```python
from build123d import *

# Parameters (mm, degrees)
SKETCH1_R           = 3.556
BOSS_EXTRUDE2_DEPTH = 6.35
SKETCH2_W           = 25.4
SKETCH2_H           = 12.7
BOSS_EXTRUDE3_DEPTH = 8.255
SKETCH3_W           = 1.27
SKETCH3_H           = 3.175
CUT_EXTRUDE1_DEPTH  = 3.175
SKETCH4_R           = 6.477
CUT_EXTRUDE2_DEPTH  = 6.604
FILLET1_R           = 8.255


with BuildPart() as part:
    # Sketch1 → Boss-Extrude2 (new body)
    with BuildSketch(Plane(origin=(0, 0, 0), x_dir=(1, 0, 0), z_dir=(0, 1, 0))):
        with BuildLine():
            Line((-12.7, 0), (-12.7, 38.1))
            Line((-12.7, 38.1), (12.7, 38.1))
            Line((12.7, 38.1), (12.7, 0))
            ThreePointArc((12.7, 0), (0, -12.7), (-12.7, 0))
        make_face()
        Circle(SKETCH1_R, mode=Mode.SUBTRACT)
    extrude(amount=BOSS_EXTRUDE2_DEPTH)

    # Sketch2 → Boss-Extrude3 (add)
    with BuildSketch(Plane.XZ):
        with Locations((0, -31.75)):
            Rectangle(SKETCH2_W, SKETCH2_H)
    extrude(amount=BOSS_EXTRUDE3_DEPTH)

    # Sketch3 → Cut-Extrude1 (cut)
    with BuildSketch(Plane.XY.offset(-25.4)):
        with Locations((0, -4.7625)):
            Rectangle(SKETCH3_W, SKETCH3_H)
    extrude(amount=-CUT_EXTRUDE1_DEPTH, mode=Mode.SUBTRACT)

    # Sketch4 → Cut-Extrude2 (cut)
    with BuildSketch(Plane(origin=(0, 0, -38.1), x_dir=(-1, 0, 0), z_dir=(0, 0, -1))):
        with Locations((0, -0.9525)):
            Circle(SKETCH4_R)
    extrude(amount=-CUT_EXTRUDE2_DEPTH, mode=Mode.SUBTRACT)

    # Fillet1
    fillet1_edges = [part.edges().sort_by_distance(p)[0] for p in [
        (-12.7, -8.255, -31.75),
        (12.7, -8.255, -31.75),
    ]]
    fillet(fillet1_edges, radius=FILLET1_R)


solid = part.part
```
CAD build for the part. Positions are in the model's coordinates, mm. A direction names the side the tool comes from. Round coordinates to 2 decimals unless told otherwise and drop trailing zeros. Order: outer loops, then holes, each group sorted by start corner. A loop starts at its lowest first (then second) coordinate and runs counter-clockwise, first axis right, second up. Notation, with made-up numbers: (-20.75, 46.5) -> (-10.75, 46.5) arc R9 cw to (-10.75, 60.5) -> close; hole circle Ø4 at (-16, -6). An arc over 180 degrees is marked (long way). Write item = value, one per line.
(1) Drill centre lines: L1, parallel to Y at x = 0.5, z = 4.5; L2, parallel to Z at x = -1.25, y = -2; L3, parallel to Z at x = 1, y = 5.5. Where is each one in solid material? Low to high.
Answers follow:
L1 = 0 to 6.35
L2 = -31.5 to -25.4
L3 = -38.1 to -3.41, 3.41 to 12.66
(2) Flat gauge pins, fed straight in: P1, Ø3.5, axis at y = -4.5, z = -27.5, coming from the +X side; P2, Ø1, axis at x = 7, z = -12.5, coming from the -Y side; P3, Ø1.6, axis at y = -5.5, z = -27.5, coming from the -X side. Where does each tip first touch, or does it go through?
Answers follow:
P1 = 12.23
P2 = 0
P3 = -11.23
(3) Pull direction X, two halves, no side cores. Call faces 1 (the cylindrical face through (10.22, -5.9, -31.66)), 2 (the cylindrical face through (-0.77, 3.13, 3.47)), 3 (the flat face through (0, 0, -7)): +X half, -X half, draft (parallel to the pull), parting line (faces both ways), or undercut.
Answers follow:
face_1 = +X half
face_2 = undercut
face_3 = draft
(4) Cut at C-C (z = 1). Write the cut outline in (x, y), plus the area to 3 significant figures.
Answers follow:
outline = (-12.66, 0) -> (-3.41, 0) -> (-3.41, 6.35) -> (-12.66, 6.35) -> close; (3.41, 0) -> (12.66, 0) -> (12.66, 6.35) -> (3.41, 6.35) -> close
area = 117 mm²
(5) 3-axis set-ups, long thin cutter, end or side, ignore diameter. For faces 4 (the flat face through (-0.635, -5, -27)), 5 (the flat face through (12.7, 3, -19)), 6 (the flat face through (0, -3, -25.4)), 7 (the flat face through (-12.7, 3, -19)), 8 (the cylindrical face through (-6.18, 0.99, -34.84)): which of +Z, -Z, +X, -X, +Y, -Y reach the whole face in a straight line?
Answers follow:
face_4 = +Z
face_5 = +Z, -Z, +X, +Y, -Y
face_6 = +Z, +X, -X, -Y
face_7 = +Z, -Z, -X, +Y, -Y
face_8 = -Z
(6) Cut at B-B (y = 4.5). Write the cut outline in (x, z).
Answers follow:
outline = (-12.7, -38.1) -> (-3.5, -38.1) -> (-3.5, -31.5) -> (3.5, -31.5) -> (3.5, -38.1) -> (12.7, -38.1) -> (12.7, 0) arc R12.7 ccw to (-12.7, 0) -> close; hole circle Ø7.11 at (0, 0)
(7) Cut at D-D (y = -5). Write the cut outline in (x, z) (3 decimals), plus the area to 3 significant figures.
Answers follow:
outline = (-11.013, -38.1) -> (-5.057, -38.1) -> (-5.057, -31.496) -> (5.057, -31.496) -> (5.057, -38.1) -> (11.013, -38.1) -> (11.013, -25.4) -> (0.635, -25.4) -> (0.635, -28.575) -> (-0.635, -28.575) -> (-0.635, -25.4) -> (-11.013, -25.4) -> close
area = 209 mm²
